Autodesk Inventor part; units mm, degrees
ref_plane "YZ Plane" through (0, 0, 0) normal (1, 0, 0) x (0, 1, 0)
ref_plane "XZ Plane" through (0, 0, 0) normal (0, 1, 0) x (-1, 0, 0)
ref_plane "XY Plane" through (0, 0, 0) normal (0, 0, 1) x (1, 0, 0)
sketch "Sketch1" plane through (0, 0, 0) normal (1, 0, 0) x (0, 1, 0)
  line L0 (-63.8691, 100.7559) -> (-60.6941, 100.7559)
  line L1 (-12.0126, 2.1649) -> (-29.1539, 76.4119)
  line L2 (-12.0126, 2.1649) -> (64.1874, 2.1649) construction
  line L3 (-12.0126, 2.1649) -> (26.0874, -63.8262)
  line L4 (-12.0126, 2.1649) -> (64.1874, 2.1649) construction
  line L5 (26.0874, -63.8262) -> (127.3008, -72.6812)
  line L6 (-29.1539, 76.4119) -> (-26.0603, 77.1261)
  line L7 (-26.0603, 77.1261) -> (-8.7541, 2.1649)
  line L8 (127.3008, -72.6812) -> (126.5865, -69.5876)
  line L9 (126.5865, -69.5876) -> (28.235, -60.983)
  line L10 (1.2031, -15.1211) -> (28.235, -60.983)
  line L11 (1.2031, -15.1211) -> (-8.7541, 2.1649)
  dimension "d4" = 3.175
  dimension "d6" = 76.2
  dimension "d7" = 103
  dimension "d8" = 76.2
  dimension "d9" = 60
  dimension "d10" = 101.6
  dimension "d11" = 125
  dimension "d12" = 3.175
  dimension "d13" = 3.175
extrude "Extrusion1" add sketch "Sketch1" along normal mid plane 165.1
sketch "Sketch2" plane through (82.55, 0, 0) normal (1, 0, 0) x (0, 0, -1)
  line L0 (63.8262, 26.0874) -> (72.6812, 127.3008)
  line L1 (69.5876, 126.5865) -> (60.983, 28.235)
  line L2 (72.6812, 127.3008) -> (-77.2337, 127.3008)
  line L3 (-77.2337, 127.3008) -> (-77.2337, -29.1539)
  line L4 (-77.2337, -29.1539) -> (-76.4119, -29.1539)
  line L5 (72.6812, 127.3008) -> (63.8262, 26.0874)
  line L6 (-76.4119, -29.1539) -> (-2.1649, -12.0126)
  line L7 (-2.1649, -12.0126) -> (63.8262, 26.0874)
  line L8 (-76.4119, -29.1539) -> (-2.1649, -12.0126)
  line L9 (-2.1649, -12.0126) -> (63.8262, 26.0874)
  point P0 (0, 0)
extrude "Extrusion2" add sketch "Sketch2" along normal blind 3.175
sketch "Sketch3" plane through (-82.55, 0, 0) normal (-1, 0, 0) x (0, 0, 1)
  line L0 (-69.5876, 126.5865) -> (-72.6812, 127.3008)
  line L1 (-72.6812, 127.3008) -> (-63.8262, 26.0874)
  line L2 (-63.8262, 26.0874) -> (2.1649, -12.0126)
  line L3 (77.2337, -29.1539) -> (-72.6812, -29.1539)
  line L4 (-72.6812, -29.1539) -> (-72.6812, 127.3008)
  line L5 (-72.6812, 127.3008) -> (77.2337, 127.3008)
  line L6 (77.2337, 127.3008) -> (77.2337, -29.1539)
  line L7 (-72.6812, 127.3008) -> (-63.8262, 26.0874)
  line L8 (-63.8262, 26.0874) -> (2.1649, -12.0126)
  line L9 (2.1649, -12.0126) -> (76.4119, -29.1539)
  line L10 (76.4119, -29.1539) -> (77.2337, -29.1539)
  point P0 (0, 0)
extrude "Extrusion3" add sketch "Sketch3" along normal blind 3.175 contours L5 L6 L3 L9 L2 L1
sketch "Sketch4" plane through (-82.55, 0, 0) normal (1, 0, 0) x (0, 0, -1)
  circle A0 centre (1.0549, 35.2051) radius 2.413
  point P0 (0, 0)
  dimension "d21" = 4.826
extrude "Extrusion4" cut sketch "Sketch4" along normal through all both and the other way through all
properties part number "Bucket"
Work out the finished part from the listing and answer in its coordinate system (mm). A direction names the side the tool comes from. Round coordinates to 2 decimals unless told otherwise and drop trailing zeros. Write each loop counter-clockwise with the first axis right and the second up, starting at its lowest first coordinate (ties: lowest second). Pieces come first, ordered by that corner, then holes.
1) A cutting plane is placed at A-A on x = 27.5. Determine the outline of the cut face in (y, z) (1 decimal).
2) Which of the six approach directions +Z, -Z, +X, -X, +Y, -Y give full straight-line access (tool end or side, diameter ignored) to faces 4 (the face through (-1.16, -17.53, 40.17)), 5 (the face through (-85.725, 68, 1))?
3) A cutting plane is placed at C-C on z = -50. Determine the outline of the cut face in (x, y) (3 decimals), and give its area (3 significant figures).
4) Determine the mould class of faces 1 (the face through (85.725, 68, 3)), 2 (the face through (84.115, 37.346, -2.168)), 3 (the face through (1.2, -20.463, 38.769)) for opening direction Z: pulls with the +Z half, pulls with the -Z half, needs draft (parallel to the pull), parting line crosses it, or undercut.
5) Flat-ended cylindrical pins translate along their axes: P1, Ø12, axis at x = -28.5, y = 18.5, coming from the +Z side; P2, Ø3, axis at x = -36, z = 9.5, coming from the -Y side; P3, Ø4, axis at x = -33.5, y = 32, coming from the +Z side. Find the tip coordinate at first contact, or state that the pin passes through.
6) A cutting plane is placed at B-B on y = 68. Determine the outline of the cut face in (x, z) (3 decimals).
7) Consider probe 1 along X at (y, z) = (17, 60.5) (3 decimals); probe 2 along Y at (x, z) = (-45, -48); probe 3 along Z at (x, y) = (30, 8). Determine where each line is inside the solid, lowest interval first.
Entries:
1. outline: (-29.2, 76.4) - (-12, 2.2) - (26.1, -63.8) - (127.3, -72.7) - (126.6, -69.6) - (28.2, -61) - (1.2, -15.1) - (-8.8, 2.2) - (-26.1, 77.1) - close
2. face 4: +Z, +Y
2. face 5: +Z, -Z, -X, +Y, -Y
3. outline: (-85.725, 18.105) - (85.725, 18.105) - (85.725, 127.301) - (82.55, 127.301) - (82.55, 21.761) - (-82.55, 21.761) - (-82.55, 127.301) - (-85.725, 127.301) - close
3. area: 1,300 mm2
4. face 1: needs draft
4. face 2: undercut
4. face 3: pulls with the -Z half
5. P1: stops at z = -34.29
5. P2: stops at y = -14.05
5. P3: stops at z = -61.14
6. outline: (-85.725, -67.493) - (85.725, -67.493) - (85.725, 77.234) - (82.55, 77.234) - (82.55, -64.462) - (-82.55, -64.462) - (-82.55, 77.234) - (-85.725, 77.234) - close
7. probe 1: x = -85.725 to -82.55, 82.55 to 85.725
7. probe 2: y = 16.95 to 20.58
7. probe 3: z = -32.5 to -26.65
